Input: part model. Units: mm. Frame: model coordinates. Give positions to 0.01 mm unless a question says otherwise; leave off trailing zeros. Answer as a JSON object with one key per item and string values. Group by question number.
(1) Material intervals for L1, parallel to Y at x = 266.5, z = 10; L2, parallel to Y at x = 85.5, z = 8; L3, parallel to Z at x = -180, y = -3.6, sorted ascending.
(2) Pin query (flat end, axial travel): P1, Ø2.5, axis at x = 0, z = 0, coming from the +Y side; P2, Ø5, axis at x = 300, z = 0, coming from the -Y side; P3, Ø5, axis at x = -360, z = 4.5, coming from the +Y side; P4, Ø2.5, axis at x = 299.5, z = 1.5, coming from the +Y side. Return the tip coordinate at first contact, or that it passes through.
(3) Mould query, pull axis Z, two halves, no side actions, for faces 1 (the flat face through (-66, -0.25, 0)), 2 (the flat face through (-66, -4.35, 0)). Classes: +Z half, -Z half, draft (parallel to the pull), parting line (faces both ways), or undercut.
```python
from build123d import *

# Parameters (mm, degrees)
BOSS_EXTRUDE1_DEPTH      = 500
BOSS_EXTRUDE1_DEPTH_BACK = 500
LPATTERN1_COUNT          = 17
LPATTERN1_PITCH          = 60
SKETCH6_W                = 123.7
SKETCH6_H                = 3.75
CUT_EXTRUDE1_DEPTH       = 501.257873501
SKETCH7_W                = 10.16
SKETCH7_H                = 57.415034805
CUT_EXTRUDE2_DEPTH       = 501.257873501
SKETCH8_W                = 13.97
SKETCH8_H                = 49.36174071
CUT_EXTRUDE3_DEPTH       = 501.257873501


with BuildPart() as part:
    # Sketch5 → Boss-Extrude1 (new, two sides: drawn at the far end of the back side and taken through both)
    with BuildSketch(Plane(origin=(0, 0, 0), x_dir=(0, 0, -1), z_dir=(1, 0, 0)).offset(-BOSS_EXTRUDE1_DEPTH_BACK)):
        with BuildLine():
            Line((8.75, 4.35), (8.75, 3.25))
            Line((8.75, 3.25), (11.5, 3.25))
            ThreePointArc((11.5, 3.25), (11.853553391, 3.103553391), (12, 2.75))
            Line((12, 2.75), (12, 0.25))
            ThreePointArc((12, 0.25), (11.853553391, -0.103553391), (11.5, -0.25))
            Line((11.5, -0.25), (7.95, -0.25))
            ThreePointArc((7.95, -0.25), (7.75, -0.45), (7.55, -0.25))
            Line((7.55, -0.25), (-7.55, -0.25))
            ThreePointArc((-7.55, -0.25), (-7.75, -0.45), (-7.95, -0.25))
            Line((-7.95, -0.25), (-11.5, -0.25))
            ThreePointArc((-11.5, -0.25), (-11.853553391, -0.103553391), (-12, 0.25))
            Line((-12, 0.25), (-12, 2.75))
            ThreePointArc((-12, 2.75), (-11.853553391, 3.103553391), (-11.5, 3.25))
            Line((-11.5, 3.25), (-8.75, 3.25))
            Line((-8.75, 3.25), (-8.75, 4.35))
            Line((-8.75, 4.35), (-12.5, 4.35))
            ThreePointArc((-12.5, 4.35), (-13.207106781, 4.057106781), (-13.5, 3.35))
            Line((-13.5, 3.35), (-13.5, -0.35))
            ThreePointArc((-13.5, -0.35), (-13.207106781, -1.057106781), (-12.5, -1.35))
            Line((-12.5, -1.35), (-7.8, -1.35))
            ThreePointArc((-7.8, -1.35), (-7.05, -2.1), (-7.8, -2.85))
            Line((-7.8, -2.85), (-10.8, -2.85))
            ThreePointArc((-10.8, -2.85), (-10.941421356, -2.908578644), (-11, -3.05))
            Line((-11, -3.05), (-11, -4.35))
            Line((-11, -4.35), (11, -4.35))
            Line((11, -4.35), (11, -3.05))
            ThreePointArc((11, -3.05), (10.941421356, -2.908578644), (10.8, -2.85))
            Line((10.8, -2.85), (7.8, -2.85))
            ThreePointArc((7.8, -2.85), (7.05, -2.1), (7.8, -1.35))
            Line((7.8, -1.35), (12.5, -1.35))
            ThreePointArc((12.5, -1.35), (13.207106781, -1.057106781), (13.5, -0.35))
            Line((13.5, -0.35), (13.5, 3.35))
            ThreePointArc((13.5, 3.35), (13.207106781, 4.057106781), (12.5, 4.35))
            Line((12.5, 4.35), (8.75, 4.35))
        make_face()
    extrude(amount=BOSS_EXTRUDE1_DEPTH + BOSS_EXTRUDE1_DEPTH_BACK)

    # Sketch3 → Cut-Revolve1 (revolve, cut)
    with BuildSketch(Plane.XY, mode=Mode.PRIVATE) as cut_revolve1_sk:
        Polygon((-484.25, 0), (-484.25, -3.35), (-482, -3.35), (-482, -4.35), (-480, -4.35), (-480, 0), align=None)
    cut_revolve1 = revolve(cut_revolve1_sk.sketch.rotate(Axis((-480, -4.35, 0), (0, 1, 0)), 270), axis=Axis((-480, -4.35, 0), (0, 1, 0)), mode=Mode.SUBTRACT)

    # LPattern1: Cut-Revolve1 ×17
    with Locations(*[(i * LPATTERN1_PITCH, 0, 0) for i in range(1, LPATTERN1_COUNT)]):
        add(cut_revolve1, mode=Mode.SUBTRACT)

    # Sketch6 → Cut-Extrude1 (cut, through all)
    with BuildSketch(Plane(origin=(0, 4.35, 0), x_dir=(1, 0, 0), z_dir=(0, 1, 0))):
        Polygon((376.3, 112.746397819), (376.3, 13.5), (376.3, 12.5), (500, 12.5), (500, 8.75), (376.3, 8.75), (376.3, -272.64081393), (559.245488979, -272.64081393), (559.245488979, 112.746397819), align=None)
        with Locations((438.15, 10.625)):
            Rectangle(SKETCH6_W, SKETCH6_H)
    extrude(amount=-CUT_EXTRUDE1_DEPTH, mode=Mode.SUBTRACT)

    # Sketch7 → Cut-Extrude2 (cut, through all)
    with BuildSketch(Plane(origin=(0, 4.35, 0), x_dir=(1, 0, 0), z_dir=(0, 1, 0))):
        with Locations((371.22, -15.207517403)):
            Rectangle(SKETCH7_W, SKETCH7_H)
    extrude(amount=-CUT_EXTRUDE2_DEPTH, mode=Mode.SUBTRACT)

    # Sketch8 → Cut-Extrude3 (cut, through all)
    with BuildSketch(Plane(origin=(0, 4.35, 0), x_dir=(1, 0, 0), z_dir=(0, 1, 0))):
        with Locations((-493.015, -11.180870355)):
            Rectangle(SKETCH8_W, SKETCH8_H)
    extrude(amount=-CUT_EXTRUDE3_DEPTH, mode=Mode.SUBTRACT)


solid = part.part
```
Recorded:
{
 "1": {"L1": "y = -4.35 to -2.85, -1.35 to -0.25, 3.25 to 4.35", "L2": "y = -4.35 to -2.85, -1.35 to -0.25", "L3": "z = -11 to -2, 2 to 11"},
 "2": {"P1": "passes through", "P2": "stops at y = -4.35", "P3": "stops at y = -0.25", "P4": "stops at y = -3.35"},
 "3": {"face 1": "undercut", "face 2": "draft"}
}
